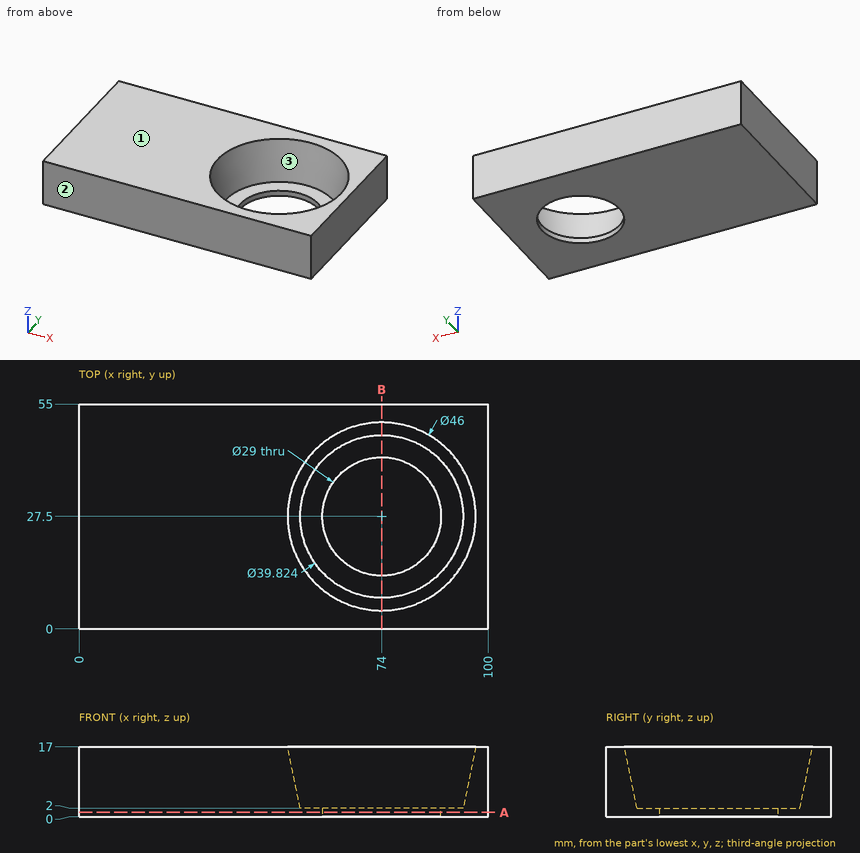
Print and shaded views of the part. All mm, measured from the part's lowest x, y and z. Coordinates: 2 decimals unless noted, no trailing zeros. Order: outer loops, then holes, each group sorted by start corner. A loop starts at its lowest first (then second) coordinate and runs counter-clockwise, first axis right, second up. Notation, with made-up numbers: (-13.75, -40) -> (8.25, -40) arc R18 ccw to (8.25, -8) -> close; hole circle Ø6 at (75, -11.75). An arc over 180 degrees is marked (long way). Answer as a JSON object with one key per item and string values. Group by question number.
1) Pull direction Y, two halves, no side cores. Call the marked faces 1, 2 and 3: +Y half, -Y half, draft (parallel to the pull), parting line (faces both ways), or undercut.
2) Cut at B-B, the plane x = 74. Write the cut outline in (y, z), then the cut area to 3 significant figures.
3) Drill centre lines: L1, parallel to Y at x = 74, z = 0.9; L2, parallel to X at y = 27.5, z = 0.7; L3, parallel to Z at x = 62.5, y = 39.5. Where is each one in solid material? Low to high.
4) Cut at A-A, the plane z = 1. Write the cut outline in (x, y).
5) Flat gauge pin, fed straight in: pin 1 (2 mm diameter, centred on x = 50, y = 23, fed in from -Z). Where does the tip first touch, or does it go through?
Check values:
{
 "1": {"face 1": "draft", "face 2": "-Y half", "face 3": "undercut"},
 "2": {"outline": "(0, 0) -> (13, 0) -> (13, 2) -> (7.59, 2) -> (4.5, 17) -> (0, 17) -> close; (42, 0) -> (55, 0) -> (55, 17) -> (50.5, 17) -> (47.41, 2) -> (42, 2) -> close", "area": "233 mm²"},
 "3": {"L1": "y = 0 to 13, 42 to 55", "L2": "x = 0 to 59.5, 88.5 to 100", "L3": "z = 0 to 2"},
 "4": {"outline": "(0, 0) -> (100, 0) -> (100, 55) -> (0, 55) -> close; hole circle Ø29 at (74, 27.5)"},
 "5": {"pin 1": "stops at z = 0"}
}
